Geometry: final body of the model. Coordinates: model frame, mm. A direction names the side the tool comes from. Give positions to 0.01 mm unless a question says otherwise; leave off trailing zeros. Write each loop counter-clockwise with the first axis right and the second up, starting at its lowest first coordinate (ties: lowest second). Pieces come first, ordered by that corner, then holes. Notation, with made-up numbers: M 11,25 L 69,25 A20 ccw 69,34 Z; hole C 89.5,-3 d10. An arc over 180 degrees is marked long. Use one line per item in the form item = value. Start each with the question number.
Item 1: Section query B-B on z = 35.5. Return loops of the section in (x, y), then the cut area to 4 significant figures.
Item 2: Section query C-C on y = 12.5. Return loops of the section in (x, z).
Item 3: Section query D-D on z = 0. Return loops of the section in (x, y).
Item 4: Access query for faces 4 (the flat face through (-30, 0, 28)), 5 (the cylindrical face through (-59.604, 85.804, -3.27)). Directions: +Z, -Z, +X, -X, +Y, -Y. A direction counts if a zero-diameter tool reaches every point of the face in a straight line with its end or side. Return the directions, or none.
Item 5: Pull-direction query (X, two-part tool) for faces 1 (the flat face through (-53, 100, -3)), 2 (the cylindrical face through (-39.79, 36.5, -1.75)), 3 (the cylindrical face through (-14.08, 35.5, 63.42)); classes: released by +X, released by -X, zero draft, split by the parting line, or undercut.
Item 6: Section query A-A on x = 0. Return loops of the section in (y, z).
Item 7: Contact query for flat-ended pins moving along their axis: P1, Ø1, axis at y = 25, z = 6.5, coming from the -X side; P2, Ø2, axis at y = 49, z = 33, coming from the -X side; P3, Ø3, axis at x = 17.5, y = 60, coming from the +Z side. Output: stop coordinate, or through.
Item 8: Material intervals for line 1 along X through (y, z) = (55, 0); line 2 along X through (y, z) = (5.5, 1), sorted ascending. Write a range as from..to.
from build123d import *

# Parameters (mm, degrees)
SKETCH1_R           = 64.964891119
BOSS_EXTRUDE1_DEPTH = 72
SKETCH2_R           = 39.826869817
CUT_EXTRUDE1_DEPTH  = 72
SKETCH3_R           = 7.132695563
BOSS_EXTRUDE2_DEPTH = 28


with BuildPart() as part:
    # Sketch1 → Boss-Extrude1 (new body)
    with BuildSketch(Plane(origin=(0, 0, 0), x_dir=(1, 0, 0), z_dir=(0, 1, 0))):
        Circle(SKETCH1_R)
    extrude(amount=BOSS_EXTRUDE1_DEPTH)

    # Sketch2 → Cut-Extrude1 (cut)
    with BuildSketch(Plane(origin=(0, 72, 0), x_dir=(1, 0, 0), z_dir=(0, 1, 0))):
        Circle(SKETCH2_R)
    extrude(amount=-CUT_EXTRUDE1_DEPTH, mode=Mode.SUBTRACT)

    # Sketch3 → Boss-Extrude2 (add)
    with BuildSketch(Plane(origin=(0, 72, 0), x_dir=(1, 0, 0), z_dir=(0, 1, 0))):
        with Locations((-52.478167306, 2.956579855)):
            Circle(SKETCH3_R)
    extrude(amount=BOSS_EXTRUDE2_DEPTH)


solid = part.part
Answer sheet:
q1.outline = M -54.41,0 L -18.05,0 L -18.05,72 L -54.41,72 Z; M 18.05,0 L 54.41,0 L 54.41,72 L 18.05,72 Z
q1.area = 5,235 mm2
q2.outline = C 0,0 d129.93; hole C 0,0 d79.65
q3.outline = M -64.96,0 L -39.83,0 L -39.83,72 L -45.99,72 L -45.99,100 L -58.97,100 L -58.97,72 L -64.96,72 Z; M 39.83,0 L 64.96,0 L 64.96,72 L 39.83,72 Z
q4.face_4 = +Z, -Z, +X, -X, -Y
q4.face_5 = +Y
q5.face_1 = zero draft
q5.face_2 = undercut
q5.face_3 = split by the parting line
q6.outline = M 0,-64.96 L 72,-64.96 L 72,-39.83 L 0,-39.83 Z; M 0,39.83 L 72,39.83 L 72,64.96 L 0,64.96 Z
q7.P1 = -64.69
q7.P2 = -56.54
q7.P3 = 62.96
q8.line_1 = -64.96..-39.83, 39.83..64.96
q8.line_2 = -64.96..-39.81, 39.81..64.96
